The listing builds one solid part. Answer for the finished solid, in the listing's coordinates (mm). A direction names the side the tool comes from. Coordinates: 2 decimals unless noted, no trailing zeros. Order: outer loops, then holes, each group sorted by start corner. A loop starts at its lowest first (then second) coordinate and runs counter-clockwise, first axis right, second up. Notation, with made-up numbers: (24.25, 30) -> (71.25, 30) arc R18 cw to (71.25, 59) -> close; hole circle Ø4 at (69.5, 46.25). An arc over 180 degrees is marked (long way). One line per question, with ' | ' between items.
from build123d import *

# Parameters (mm, degrees)
CROQUIS2_W              = 30
CROQUIS2_H              = 60
SALIENTE_EXTRUIR1_DEPTH = 6
REDONDEO1_R             = 10
REDONDEO2_R             = 10
CROQUIS3_R              = 1.35
CORTAR_EXTRUIR1_DEPTH   = 7
CORTAR_EXTRUIR2_DEPTH   = 2


with BuildPart() as part:
    # Croquis2 → Saliente-Extruir1 (new body)
    with BuildSketch(Plane(origin=(0, 0, 0), x_dir=(1, 0, 0), z_dir=(0, 1, 0))):
        with Locations((0, 30)):
            Rectangle(CROQUIS2_W, CROQUIS2_H)
        with BuildLine():
            Line((-5.5, 35), (-5.5, 10))
            ThreePointArc((-5.5, 10), (-7.5, 8), (-9.5, 10))
            Line((-9.5, 10), (-9.5, 35))
            ThreePointArc((-9.5, 35), (-7.5, 37), (-5.5, 35))
        make_face(mode=Mode.SUBTRACT)
        with BuildLine():
            Line((9.5, 35), (9.5, 10))
            ThreePointArc((9.5, 10), (7.5, 8), (5.5, 10))
            Line((5.5, 10), (5.5, 35))
            ThreePointArc((5.5, 35), (7.5, 37), (9.5, 35))
        make_face(mode=Mode.SUBTRACT)
        with BuildLine():
            Line((3, 35), (3, 25))
            ThreePointArc((3, 25), (0, 22), (-3, 25))
            Line((-3, 25), (-3, 35))
            ThreePointArc((-3, 35), (0, 38), (3, 35))
        make_face(mode=Mode.SUBTRACT)
    extrude(amount=SALIENTE_EXTRUIR1_DEPTH)

    # Redondeo1
    redondeo1_edges = [part.edges().sort_by_distance(p)[0] for p in [
        (-15, 3, -60),
        (15, 3, -60),
    ]]
    fillet(redondeo1_edges, radius=REDONDEO1_R)

    # Redondeo2
    redondeo2_edges = [part.edges().sort_by_distance(p)[0] for p in [
        (15, 3, 0),
        (-15, 3, 0),
    ]]
    fillet(redondeo2_edges, radius=REDONDEO2_R)

    # Croquis3 → Cortar-Extruir1 (cut, through all)
    with BuildSketch(Plane.XZ):
        with Locations((4.75, -52.7)):
            Circle(CROQUIS3_R)
        with Locations((-4.75, -52.7)):
            Circle(CROQUIS3_R)
    extrude(amount=-CORTAR_EXTRUIR1_DEPTH, mode=Mode.SUBTRACT)

    # Croquis4 → Cortar-Extruir2 (cut)
    with BuildSketch(Plane(origin=(0, 6, 0), x_dir=(-1, 0, 0), z_dir=(0, -1, 0))):
        Polygon((-2.1, 51.170021787), (-2.1, 54.229978213), (-4.75, 55.759956427), (-7.4, 54.229978213), (-7.4, 51.170021787), (-4.75, 49.640043573), align=None)
        Polygon((7.4, 51.170021787), (7.4, 54.229978213), (4.75, 55.759956427), (2.1, 54.229978213), (2.1, 51.170021787), (4.75, 49.640043573), align=None)
    extrude(amount=CORTAR_EXTRUIR2_DEPTH, mode=Mode.SUBTRACT)


solid = part.part
Item 1: Find the intervals of material crossed by L1, parallel to X at y = 2.25, z = -13; L2, parallel to Z at x = 4.75, y = 1.45; L3, parallel to Y at x = -4.5, z = -50.5, in increasing order.
Computed values:
L1: x = -15 to -9.5, -5.5 to 5.5, 9.5 to 15 | L2: z = -60 to -54.05, -51.35 to 0 | L3: y = 0 to 4
Item 2: Each of these flat-tipped pins is pushed along its axis until it touches: pin 1 Ø3 at (x, z) = (-4.75, -52.7) entering from +Y; pin 2 Ø1.6 at (y, z) = (5, -53.5) entering from -X; pin 3 Ø0.6 at (y, z) = (5, -52) entering from +X; pin 4 Ø6 at (x, z) = (-4.5, -52) entering from +Y. Where does it stop, or does it pass through?
Computed values:
pin 1: stops at y = 4 | pin 2: stops at x = -14.63 | pin 3: stops at x = 14.85 | pin 4: stops at y = 6
Item 3: Section A-A, the plane x = 0 is taken. Give the vertices of the cut face in (y, z), plus the area to 3 significant figures.
Computed values:
outline: (0, -60) -> (6, -60) -> (6, -38) -> (0, -38) -> close; (0, -22) -> (6, -22) -> (6, 0) -> (0, 0) -> close | area: 264 mm^2
Item 4: Section B-B, the plane z = -27 is taken. Give the vertices of the cut face in (x, y).
Computed values:
outline: (-15, 0) -> (-9.5, 0) -> (-9.5, 6) -> (-15, 6) -> close; (-5.5, 0) -> (-3, 0) -> (-3, 6) -> (-5.5, 6) -> close; (3, 0) -> (5.5, 0) -> (5.5, 6) -> (3, 6) -> close; (9.5, 0) -> (15, 0) -> (15, 6) -> (9.5, 6) -> close
Item 5: For faces 1 (the face through (-6.094, 5.014, -54.984)), 2 (the face through (3, 3, -30)), 3 (the face through (0, 3, -60)), determine the directions among +Z, -Z, +X, -X, +Y, -Y from which every point of the face is accessible in a straight line to the end or side of a thin tool.
Computed values:
face 1: +Y | face 2: +Y, -Y | face 3: -Z, +X, -X, +Y, -Y
Item 6: Section D-D, the plane z = -15.5 is taken. Give the vertices of the cut face in (x, y).
Computed values:
outline: (-15, 0) -> (-9.5, 0) -> (-9.5, 6) -> (-15, 6) -> close; (-5.5, 0) -> (5.5, 0) -> (5.5, 6) -> (-5.5, 6) -> close; (9.5, 0) -> (15, 0) -> (15, 6) -> (9.5, 6) -> close
Item 7: Determine the mould class of faces 4 (the face through (-5.5, 3, -23)), 5 (the face through (-4, 0, -30)), 6 (the face through (-12.15, 3.04, -56.99)) for opening direction Z: pulls with the +Z half, pulls with the -Z half, needs draft (parallel to the pull), parting line crosses it, or undercut.
Computed values:
face 4: undercut | face 5: needs draft | face 6: pulls with the -Z half
Item 8: Section C-C, the plane y = 3 is taken. Give the vertices of the cut face in (x, z).
Computed values:
outline: (-15, -50) arc R10 ccw to (-5, -60) -> (5, -60) arc R10 ccw to (15, -50) -> (15, -10) arc R10 ccw to (5, 0) -> (-5, 0) arc R10 ccw to (-15, -10) -> close; hole (-9.5, -35) arc R2 ccw to (-5.5, -35) -> (-5.5, -10) arc R2 ccw to (-9.5, -10) -> close; hole circle Ø2.7 at (-4.75, -52.7); hole (-3, -35) arc R3 ccw to (3, -35) -> (3, -25) arc R3 ccw to (-3, -25) -> close; hole circle Ø2.7 at (4.75, -52.7); hole (5.5, -35) arc R2 ccw to (9.5, -35) -> (9.5, -10) arc R2 ccw to (5.5, -10) -> close
